from build123d import *

# Parameters (mm, degrees)
SKETCH1_R           = 1.5
SKETCH1_R_2         = 1.45
BOSS_EXTRUDE1_DEPTH = 1.5
FILLET1_R           = 20


with BuildPart() as part:
    # Sketch1 → Boss-Extrude1 (new body, symmetric)
    with BuildSketch(Plane(origin=(0, 0, 0), x_dir=(0, 0, -1), z_dir=(1, 0, 0))):
        with BuildLine():
            Line((-127.350956164, -7.122008503), (-105, -14.5))
            Line((-105, -14.5), (-13.675, -14.5))
            Line((-13.675, -14.5), (0, -12.5))
            ThreePointArc((0, -12.5), (12.276307634, 2.354202809), (-4.624146867, 11.613236661))
            Line((-4.624146867, 11.613236661), (-25, 3.5))
            Line((-25, 3.5), (-100, 3.5))
            Line((-100, 3.5), (-117.5, 7.5))
            Line((-117.5, 7.5), (-125, 7.5))
            ThreePointArc((-125, 7.5), (-132.404899181, 1.190574699), (-127.350956164, -7.122008503))
        make_face()
        with Locations((-97.5, -5.5)):
            Circle(SKETCH1_R, mode=Mode.SUBTRACT)
        Polygon((-89.5, -7), (-89.5, -4), (-88, -2.5), (-29.5, -2.5), (-28, -4), (-28, -7), (-29.5, -8.5), (-88, -8.5), align=None, mode=Mode.SUBTRACT)
        with Locations((-20, -5.5)):
            Circle(SKETCH1_R, mode=Mode.SUBTRACT)
        with Locations((-125, 0)):
            Circle(SKETCH1_R_2, mode=Mode.SUBTRACT)
        Circle(SKETCH1_R_2, mode=Mode.SUBTRACT)
    extrude(amount=BOSS_EXTRUDE1_DEPTH, both=True)

    # Fillet1
    fillet1_edges = [part.edges().sort_by_distance(p)[0] for p in [
        (0, -14.5, 105),
        (0, 7.5, 117.5),
        (0, 3.5, 100),
        (0, 3.5, 25),
    ]]
    fillet(fillet1_edges, radius=FILLET1_R)


solid = part.part
Geometry check sheet. Reference: the model listing, model coordinates, mm. A direction names the side the tool comes from. Coordinates: 2 decimals unless noted, no trailing zeros. Order: outer loops, then holes, each group sorted by start corner. A loop starts at its lowest first (then second) coordinate and runs counter-clockwise, first axis right, second up. Notation, with made-up numbers: M 33.25,77 L 40.25,77 A20 cw 40.25,108 Z; hole C -36.5,85.25 d7. An arc over 180 degrees is marked long. Use CSV: the item, a comma, the result in double quotes.
Item 1: Cross-section at A-A on x = 0. Record the cut outline in (y, z) (3 decimals), then the cut area to 3 significant figures.
Returned:
outline,"M -14.5,13.675 L -12.5,0 A12.5 ccw long 11.613,4.624 L 4.919,21.437 A20 cw 3.5,28.835 L 3.5,97.743 A20 cw 4.003,102.2 L 6.997,115.3 A20 ccw 7.5,119.757 L 7.5,125 A7.5 ccw -7.122,127.351 L -13.492,108.054 A20 ccw -14.5,101.784 Z; hole M -8.5,29.5 L -7,28 L -4,28 L -2.5,29.5 L -2.5,88 L -4,89.5 L -7,89.5 L -8.5,88 Z; hole C -5.5,20 d3; hole C -5.5,97.5 d3; hole C 0,0 d2.9; hole C 0,125 d2.9"
area,"2,300 mm2"
Item 2: Mould release check, pull along Y, two halves, no side actions. Record for faces 6 (the cylindrical face through (-0.02, 3.85, 25.12)), 7 (the flat face through (0, -5, 28)), 8 (the flat face through (-1.5, -1, 61)): pulls with the +Y half, pulls with the -Y half, needs draft (parallel to the pull), parting line crosses it, or undercut.
Returned:
face 6,"pulls with the +Y half"
face 7,"undercut"
face 8,"needs draft"
Item 3: Cross-section at B-B on y = 0. Record the cut outline in (x, z), then the cut area to 3 significant figures.
Returned:
outline,"M -1.5,-12.5 L 1.5,-12.5 L 1.5,-1.45 L -1.5,-1.45 Z; M -1.5,1.45 L 1.5,1.45 L 1.5,123.55 L -1.5,123.55 Z; M -1.5,126.45 L 1.5,126.45 L 1.5,132.5 L -1.5,132.5 Z"
area,"418 mm2"
Item 4: Thickness scan on line 1 along Y through (x, z) = (-0.8, 97.5); line 2 along Y through (x, z) = (0.6, 61); line 3 along Z through (x, y) = (-1.25, -2.75). Record the ranges inside material, lowest first.
Returned:
line 1,"y = -14.5 to -7, -4 to 3.5"
line 2,"y = -14.5 to -8.5, -2.5 to 3.5"
line 3,"z = -12.19 to 29.25, 88.25 to 131.98"
Item 5: Gauge pin test, flat ends, axial feed: pin 1 Ø5 at (y, z) = (-5.5, 20) entering from +X; pin 2 Ø1.5 at (x, z) = (0.5, 56.5) entering from +Y; pin 3 Ø1.5 at (x, z) = (-0.5, 2.5) entering from -Y; pin 4 Ø0.9 at (x, z) = (-0.5, 121) entering from +Y. Record the tip position at first contact, or that the pin passes through.
Returned:
pin 1,"stops at x = 1.5"
pin 2,"stops at y = 3.5"
pin 3,"stops at y = -12.98"
pin 4,"stops at y = 7.5"
Item 6: Cross-section at D-D on y = -5.5. Record the cut outline in (x, z).
Returned:
outline,"M -1.5,-11.22 L 1.5,-11.22 L 1.5,18.5 L -1.5,18.5 Z; M -1.5,21.5 L 1.5,21.5 L 1.5,28 L -1.5,28 Z; M -1.5,89.5 L 1.5,89.5 L 1.5,96 L -1.5,96 Z; M -1.5,99 L 1.5,99 L 1.5,130.1 L -1.5,130.1 Z"
Item 7: Tool access check on faces 1 (the flat face through (0.02, 5.48, 108.66)), 2 (the flat face through (0.021, -13.514, 6.933)), 3 (the flat face through (0, -8.5, 58)), 4 (the cylindrical face through (0.02, -14.24, 105)), 5 (the flat face through (0, 7.5, 122)). Record the directions out of +Z, -Z, +X, -X, +Y, -Y that give a thin tool (end or side, any length) a straight path to the whole face; none if there is none.
Returned:
face 1,"+X, -X, +Y"
face 2,"-Z, +X, -X, -Y"
face 3,"+X, -X"
face 4,"+Z, +X, -X, -Y"
face 5,"+Z, +X, -X, +Y"
Item 8: Cross-section at C-C on z = 78.5. Record the cut outline in (x, y).
Returned:
outline,"M -1.5,-14.5 L 1.5,-14.5 L 1.5,-8.5 L -1.5,-8.5 Z; M -1.5,-2.5 L 1.5,-2.5 L 1.5,3.5 L -1.5,3.5 Z"
